Geometry check sheet. Reference: the model listing, model coordinates, mm. Face numbers are marked on the shaded views. A direction names the side the tool comes from. Round coordinates to 2 decimals unless told otherwise and drop trailing zeros. Write each loop counter-clockwise with the first axis right and the second up, starting at its lowest first coordinate (ties: lowest second). Pieces come first, ordered by that corner, then holes. Notation, with made-up numbers: (77.5, 81) - (81.5, 81) arc R17 cw to (81.5, 89) - close; hole circle Ø5 at (-6, -14.75). An arc over 180 degrees is marked (long way). Return JSON: item names as keys, results as strings.
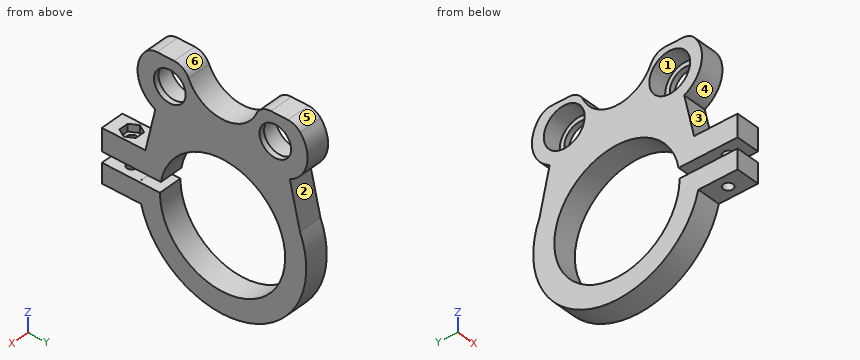
Autodesk Inventor part; units mm, degrees
sketch "Boceto1" plane through (0, 0, 0) normal (1, 0, 0) x (0, 1, 0)
  circle A0 centre (0, 0) radius 23.75
  arc A1 (-29.376, 12.0463) -> (29.376, 12.0463) centre (0, 0) ccw
  line L0 (-29.376, 12.0463) -> (-25.5135, 29.0609)
  line L1 (29.376, 12.0463) -> (25.5135, 29.0609)
  circle A2 centre (-20, 40) radius 7.75
  circle A3 centre (20, 40) radius 7.75
  arc A4 (-12.8312, 46.4) -> (12.8312, 46.4) centre (0, 52) ccw
  line L2 (-24.8023, 50) -> (-18.3303, 50)
  arc A5 (-29.4126, 47.84) -> (-25.5135, 29.0609) centre (-20, 40) ccw
  arc A6 (25.5135, 29.0609) -> (29.4126, 47.84) centre (20, 40) ccw
  line L3 (18.3303, 50) -> (24.8023, 50)
  arc A7 (18.3303, 50) -> (12.8312, 46.4) centre (18.3303, 44) ccw
  arc A8 (-12.8312, 46.4) -> (-18.3303, 50) centre (-18.3303, 44) ccw
  arc A9 (-24.8023, 50) -> (-29.4126, 47.84) centre (-24.8023, 44) ccw
  arc A10 (29.4126, 47.84) -> (24.8023, 50) centre (24.8023, 44) ccw
  point P0 (-27.0755, 50)
  point P1 (-32.25, 40)
  point P2 (32.25, 40)
  point P3 (-27.75, 40)
  point P4 (27.75, 40)
  point P5 (-13.8564, 50)
  point P6 (13.8564, 50)
  point P7 (0, 38)
  point P8 (27.0755, 50)
  dimension "d4" = 15.5
  dimension "d5" = 15.5
  dimension "d0" = 47.5
  dimension "d1" = 63.5
  dimension "d2" = 25.58
  dimension "d7" = 4.5
  dimension "d8" = 4.5
  dimension "d25" = 51.027
  dimension "d55" = 10
  dimension "d58" = 40
  dimension "d59" = 20
  dimension "d60" = 40
  dimension "d61" = 52
  dimension "d62" = 14
  dimension "d63" = 6
  dimension "d64" = 6
extrude "Extrusión1" add sketch "Boceto1" along normal blind 9
sketch "Boceto2" plane through (9, 0, 0) normal (1, 0, 0) x (0, 0, -1)
  arc A0 (-12.0463, -29.376) -> (-12.0463, 29.376) centre (0, 0) ccw
  circle A1 centre (0, 0) radius 23.75
  line L0 (7.4, -22.5677) -> (7.4, -45.7498)
  line L1 (7.4, -45.7498) -> (-0.1, -45.7498)
  line L2 (-0.1, -45.7498) -> (-0.1, -23.7498)
  circle A2 centre (0, 0) radius 23.75
  line L3 (-4.1, -23.3934) -> (-4.1, -45.7498)
  line L4 (-4.1, -45.7498) -> (-12.6, -45.7498)
  line L5 (-12.6, -45.7498) -> (-12.6, -20.1321)
  line L6 (-50, -18.3303) -> (-50, -24.8023)
  point P0 (-50, -15.6404)
  point P1 (-50, -27.0755)
  point P2 (-29.0609, -25.5135)
  dimension "d17" = 8.5
  dimension "d18" = 7.5
  dimension "d19" = 4
  dimension "d26" = 22
  dimension "d27" = 37.4
extrude "Extrusión2" add sketch "Boceto2" against normal blind 9 contours L3 L4 L5 A1 | L2 A1 L0 A0 | A0 L0 L1 L2
sketch "Boceto3" plane through (9, 0, 0) normal (1, 0, 0) x (0, 0, -1)
  circle A0 centre (-40, -20) radius 7.75
  circle A1 centre (-40, 20) radius 7.75
  circle A2 centre (-40, -20) radius 6
  circle A3 centre (-40, 20) radius 6
  point P0 (0, 0)
  dimension "d31" = 12
  dimension "d32" = 12
extrude "Extrusión3" add sketch "Boceto3" against normal blind 2
sketch "Boceto4" plane through (9, -45.7498, -7.4) normal (0, 0, -1) x (-1, 0, 0)
  line L0 (0, 0) -> (9, 0)
  line L1 (9, 14.8742) -> (9, 0)
  point P0 (9, 45.7498)
  point P1 (4.5, 7.4371)
  point P2 (4.5, 0)
  point P3 (9, 7.4371)
hole "Agujero1" at (4.5, -38.3127, -7.4) direction (0, 0, 1) diameter 3.75 end through all
sketch "Boceto5" plane through (9, -45.7498, 12.6) normal (0, 0, 1) x (1, 0, 0)
  circle A0 centre (-4.5, 7.4371) radius 1.875
  line L0 (-6.2999, 10.5546) -> (-2.7001, 10.5546)
  line L1 (-2.7001, 10.5546) -> (-0.9002, 7.4371)
  line L2 (-0.9002, 7.4371) -> (-2.7001, 4.3196)
  line L3 (-2.7001, 4.3196) -> (-6.2999, 4.3196)
  line L4 (-6.2999, 4.3196) -> (-8.0998, 7.4371)
  line L5 (-8.0998, 7.4371) -> (-6.2999, 10.5546)
  point P0 (-9, 45.7498)
  dimension "d44" = 6.235
extrude "Extrusión4" cut sketch "Boceto5" against normal blind 2.8
sketch "Boceto6" plane through (0, 0, 0) normal (-1, 0, 0) x (0, 0, 1)
  line L0 (0.1, -45.7498) -> (0.1, -31.7498)
  line L1 (4.1, -31.4842) -> (4.1, -45.7498)
  line L2 (0.1, -31.7498) -> (4.1, -31.7498)
  line L3 (4.1, -31.7498) -> (4.1, -21.7498)
  line L4 (4.1, -21.7498) -> (0.1, -21.7498)
  line L5 (0.1, -21.7498) -> (0.1, -31.7498)
  point P0 (0, 0)
  dimension "d50" = 10
extrude "Extrusión5" cut sketch "Boceto6" against normal through all
equation "\"d5\" = d4"
properties part number "G004164_Cycl_carroZ_inferior"
(1) Section check A-A, the plane y = 0. Enter the section's corners in (x, z).
Response values:
{"outline": "(0, -31.75) - (9, -31.75) - (9, -23.75) - (0, -23.75) - close; (0, 23.75) - (9, 23.75) - (9, 38) - (0, 38) - close"}
(2) Material ranges on line 1 along Z through (x, y) = (7, -40); line 2 along Y through (x, z) = (8.2, 40); line 3 along Z through (x, y) = (1.5, -20), recorded low to high. Write a range as [from, to].
Response values:
{"line 1": "z = [-7.4, 0.1], [4.1, 9.8]", "line 2": "y = [-32.25, -26], [-14, -7.21], [7.21, 14], [26, 32.25]", "line 3": "z = [-24.66, -12.81], [12.81, 32.25], [47.75, 50]"}
(3) Access from +Z, -Z, +X, -X, +Y, -Y to the whole of each face (thin tool, end or side, straight path). Record for the marked faces 1, 2 and 3.
Response values:
{"face 1": "-X", "face 2": "+X, -X, +Y", "face 3": "+X, -X, -Y"}
(4) Section check B-B, the plane z = -19.5. Enter the section's corners in (x, y).
Response values:
{"outline": "(0, -25.06) - (9, -25.06) - (9, -13.56) - (0, -13.56) - close; (0, 13.56) - (9, 13.56) - (9, 25.06) - (0, 25.06) - close"}
(5) Section check D-D, the plane x = 4.5. Give the number of separate pieces and of enclosed holes in the cut face, plus the area to 3 significant figures.
Response values:
{"separate pieces": "3", "enclosed holes": "2", "area": "2,270 mm^2"}
(6) Release check for a two-part mould opening along Y. For the marked faces 4, 5 and 6 record: pulls with the +Y half, pulls with the -Y half, needs draft (parallel to the pull), parting line crosses it, or undercut.
Response values:
{"face 4": "pulls with the -Y half", "face 5": "pulls with the +Y half", "face 6": "undercut"}
(7) Section check C-C, the plane y = -20. Enter the section's corners in (x, z), plus the area to 3 significant figures.
Response values:
{"outline": "(0, -24.66) - (9, -24.66) - (9, -12.81) - (0, -12.81) - close; (0, 12.81) - (9, 12.81) - (9, 34) - (7, 34) - (7, 32.25) - (0, 32.25) - close; (0, 47.75) - (7, 47.75) - (7, 46) - (9, 46) - (9, 50) - (0, 50) - close", "area": "309 mm^2"}
(8) Gauge pin test, flat ends, axial feed: pin 1 (2.5 mm diameter, centred on x = 5, y = -35, fed in from +Z); pin 2 (2 mm diameter, centred on x = 7.5, y = -27, fed in from -Z); pin 3 (5 mm diameter, centred on x = 1, y = 23.5, fed in from -Z); pin 4 (9.5 mm diameter, centred on y = 20, z = 40, fed in from -X). Record the tip position at first contact, or that the pin passes through.
Response values:
{"pin 1": "stops at z = 12.6", "pin 2": "stops at z = -18.22", "pin 3": "stops at z = -23.81", "pin 4": "passes through"}
